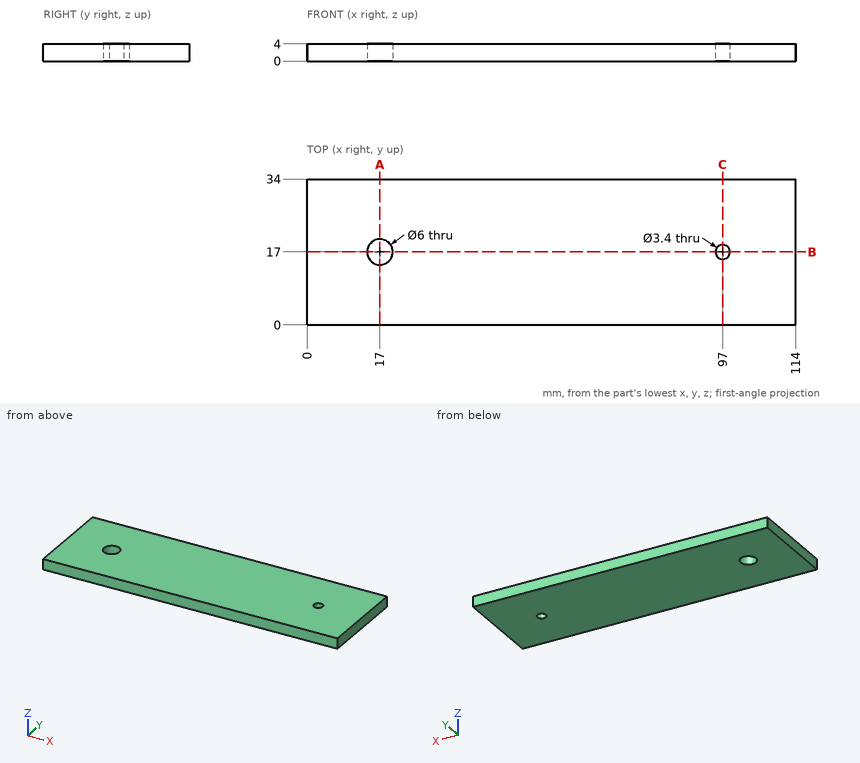
Could you check a few things on this drawing? It's one solid part, dimensions in mm from its lowest x, y, z. Round coordinates to 2 decimals unless told otherwise and drop trailing zeros. Loops run counter-clockwise (first coordinate to the right, second up) from the corner with the lowest first, then second, coordinate; pieces in that order, holes last.
Q1. I want a section at C-C (x = 97). Write out the boundary of the cut face in (y, z), and give its area (3 significant figures).
Q2. Please list where these lines run through material, in increasing order: L1, parallel to Y at x = 97, z = 1.65; L2, parallel to Y at x = 17, z = 1.5.
Q3. I want a section at A-A (x = 17). Write out the boundary of the cut face in (y, z), and give its area (3 significant figures).
Q4. I want a section at B-B (y = 17). Write out the boundary of the cut face in (x, z), and give its area (3 significant figures).
Q5. For P1, Ø1, axis at y = 18.5, z = 3.5, coming from the -X side, with a flat end and sliding along its axis, tell me the tip position at first contact or that it passes through.
Answer below:
1. outline: (0, 0) - (15.3, 0) - (15.3, 4) - (0, 4) - close; (18.7, 0) - (34, 0) - (34, 4) - (18.7, 4) - close
1. area: 122 mm2
2. L1: y = 0 to 15.3, 18.7 to 34
2. L2: y = 0 to 14, 20 to 34
3. outline: (0, 0) - (14, 0) - (14, 4) - (0, 4) - close; (20, 0) - (34, 0) - (34, 4) - (20, 4) - close
3. area: 112 mm2
4. outline: (0, 0) - (14, 0) - (14, 4) - (0, 4) - close; (20, 0) - (95.3, 0) - (95.3, 4) - (20, 4) - close; (98.7, 0) - (114, 0) - (114, 4) - (98.7, 4) - close
4. area: 418 mm2
5. P1: stops at x = 0
